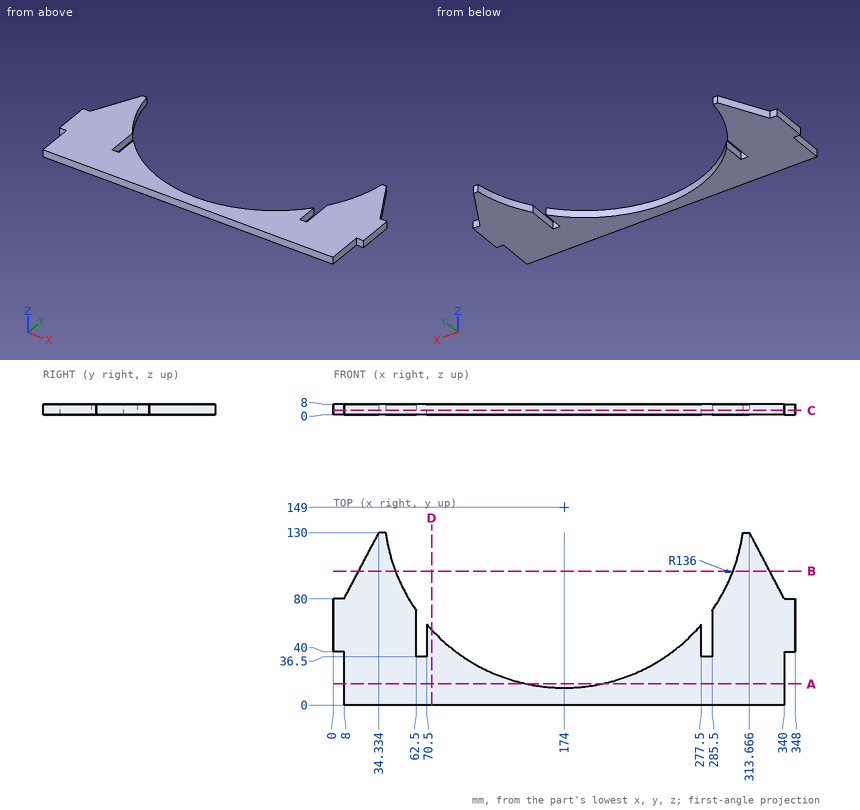
For this review, use the dimensioned drawing (mm, ordinates from the lowest corner) and the shaded views. Give positions to 0.01 mm unless a question says otherwise; leave off trailing zeros. Order: outer loops, then holes, each group sorted by start corner. A loop starts at its lowest first (then second) coordinate and runs counter-clockwise, first axis right, second up.
1. Add section C-C, the plane z = 3.25. State the section outline as (x, y) points (1 decimal).
Solution:
outline: (0, 40) - (8, 40) - (8, 0) - (340, 0) - (340, 40) - (348, 40) - (348, 80) - (340, 80) - (313.7, 130) - (308.7, 130) arc R136 cw to (285.5, 71.1) - (285.5, 36.5) - (277.5, 36.5) - (277.5, 60.8) arc R136 cw to (70.5, 60.8) - (70.5, 36.5) - (62.5, 36.5) - (62.5, 71.1) arc R136 cw to (39.3, 130) - (34.3, 130) - (8, 80) - (0, 80) - close
2. Add section D-D, the plane x = 74. State the section outline as (y, z) points, then the cut area to 3 significant figures.
Solution:
outline: (0, 0) - (56.83, 0) - (56.83, 8) - (0, 8) - close
area: 455 mm2
3. For pin 1 Ø4 at (x, z) = (342.5, 5) entering from +Y; pin 2 Ø4 at (x, z) = (343.5, 2.5) entering from -Y; pin 3 Ø4 at (x, z) = (67.5, 3.5) entering from +Y, all flat-tipped, find the tip position at first contact; note any pin that passes through.
Solution:
pin 1: stops at y = 80
pin 2: stops at y = 40
pin 3: stops at y = 36.5
4. Add section B-B, the plane y = 101. State the section outline as (x, z) points.
Solution:
outline: (19.06, 0) - (46.75, 0) - (46.75, 8) - (19.06, 8) - close; (301.25, 0) - (328.94, 0) - (328.94, 8) - (301.25, 8) - close
5. To check wall thickness, follow L1, parallel to X at y = 57.5, z = 1.75; L2, parallel to X at y = 46.5, z = 3.5 (1 decimal); L3, parallel to X at y = 89, z = 4.25. State the ranges of each line that lie inside material, in increasing order.
Solution:
L1: x = 0 to 62.5, 70.5 to 73.38, 274.62 to 277.5, 285.5 to 348
L2: x = 0 to 62.5, 70.5 to 84.6, 263.4 to 277.5, 285.5 to 348
L3: x = 12.74 to 51.95, 296.05 to 335.26
6. Add section A-A, the plane y = 16. State the section outline as (x, z) points, then the cut area to 3 significant figures.
Solution:
outline: (8, 0) - (145.59, 0) - (145.59, 8) - (8, 8) - close; (202.41, 0) - (340, 0) - (340, 8) - (202.41, 8) - close
area: 2,200 mm2
